For this review, take the finished solid that the model builds, in its own axes (mm). Face numbers are marked on the shaded views. A direction names the side the tool comes from. Coordinates: 2 decimals unless noted, no trailing zeros. Order: outer loops, then holes, each group sorted by start corner. A loop starts at its lowest first (then second) coordinate and runs counter-clockwise, first axis right, second up. Notation, with made-up numbers: (75.5, 65.5) - (109.5, 65.5) arc R20 cw to (109.5, 86.5) - close; hole circle Ø6 at (-35.5, -29.5). An arc over 180 degrees is marked (long way). One line per item, written item: value. Start each with the question number.
(1) Consider section A-A on x = 0. Write out the cut boundary in (y, z), then the cut area to 3 significant figures.
(2) For the marked faces 1, 2, 3, 4 and 5, list the 3-axis set-ups (+Z, -Z, +X, -X, +Y, -Y) from which the entire face can be reached by the end or side of a thin tool; tool diameter is ignored.
(3) To check wall thickness, follow line 1 along X through (y, z) = (-15, -4.5); line 2 along Y through (x, z) = (4.25, 0); line 3 along Z through (x, y) = (1.25, -10). State the ranges of each line that lie inside material, in increasing order.
(4) Clearance check with flat-ended pins moving along their axes: pin 1 (3 mm diameter, centred on y = -7.5, z = 0, fed in from -X); pin 2 (5 mm diameter, centred on x = 3, y = -10, fed in from +Z); pin 3 (5 mm diameter, centred on x = 3.5, y = -1, fed in from +Z). State where each tip first meets the part, or that it passes through.
(5) Consider section B-B on z = 0. Write out the cut boundary in (x, y).
(6) Consider section D-D on y = -11.5. Write out the cut boundary in (x, z), then the cut area to 3 significant figures.
(7) Mouldability with a two-part tool opening along Y and no side actions: class the marked faces 6, 7 and 8 as released by +Y, released by -Y, zero draft, split by the parting line, or undercut.
(8) Consider section C-C on y = -15. Write out the cut boundary in (x, z).
```python
from build123d import *

# Parameters (mm, degrees)
F0_R     = 5
F1_DEPTH = 1
F2_R     = 4
F3_DEPTH = 16
F4_R     = 1.5
F5_DEPTH = 5


with BuildPart() as f1:
    # F0 (on Front) → F1 (new body, symmetric)
    with BuildSketch(Plane.XZ):
        Circle(F0_R)
    extrude(amount=F1_DEPTH, both=True)

    # F2 (on face) → F3 (join)
    with BuildSketch(Plane.XZ.offset(1)):
        Circle(F2_R)
    extrude(amount=F3_DEPTH)

    # F4 (on Top) → F5 (join, symmetric)
    with BuildSketch(Plane.XY):
        with Locations((0, -15)):
            Circle(F4_R)
    extrude(amount=F5_DEPTH, both=True)


solid = f1.part
```
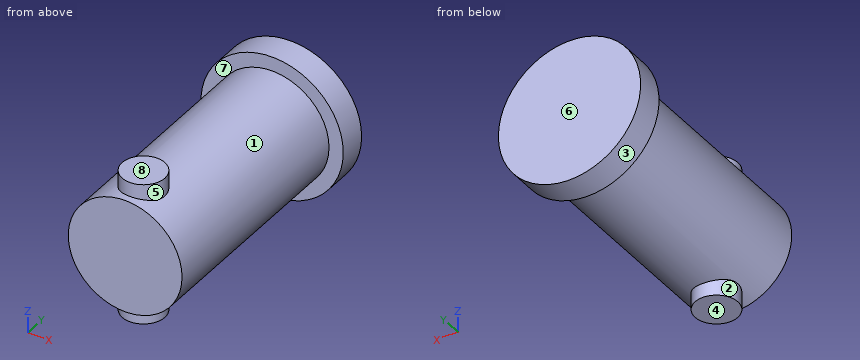
Geometry check:
1. outline: (-17, -4) - (-16.5, -4) - (-16.5, -5) - (-13.5, -5) - (-13.5, -4) - (-1, -4) - (-1, -5) - (1, -5) - (1, 5) - (-1, 5) - (-1, 4) - (-13.5, 4) - (-13.5, 5) - (-16.5, 5) - (-16.5, 4) - (-17, 4) - close
1. area: 154 mm^2
2. face 1: none
2. face 2: -Z
2. face 3: +Y
2. face 4: -Z, +X, -X, +Y, -Y
2. face 5: +Z
3. line 1: x = -1.5 to 1.5
3. line 2: y = -1 to 1
3. line 3: z = -3.8 to 3.8
4. pin 1: stops at x = -4
4. pin 2: stops at z = 3.97
4. pin 3: stops at z = 4.9
5. outline: (-5, -1) - (-4, -1) - (-4, -17) - (4, -17) - (4, -1) - (5, -1) - (5, 1) - (-5, 1) - close
6. outline: circle Ø8 at (0, 0)
6. area: 50.3 mm^2
7. face 6: released by +Y
7. face 7: undercut
7. face 8: zero draft
8. outline: (-1.5, -5) - (1.5, -5) - (1.5, -3.71) arc R4 ccw to (1.5, 3.71) - (1.5, 5) - (-1.5, 5) - (-1.5, 3.71) arc R4 ccw to (-1.5, -3.71) - close
